Here's how the part is built. I have some questions about the finished solid (model axes, mm). Face numbers are marked on the shaded views. Give positions to 0.01 mm unless a question says otherwise; leave off trailing zeros. Loops run counter-clockwise (first coordinate to the right, second up) from the corner with the lowest first, then second, coordinate; pieces in that order, holes last.
Q1. Suppose I cut it at C-C (z = -36.5). Count the separate pieces of the cut face and the enclosed holes in it, and give its area (3 significant figures).
Q2. I need wall thicknesses on probe 1 along X at (y, z) = (-31, -40); probe 2 along X at (y, z) = (-8, -39); probe 3 along Z at (x, y) = (-44, -44.5). Which ranges of each line are inside material? Lowest first, please.
Q3. Suppose I cut it at A-A (y = -25). List the corners of the cut face in (x, z) for me.
Q4. Thinking about a two-plate mould opening in X: for the marked faces 1 and 2, which applies, pulls with the +X half, pulls with the -X half, needs draft (parallel to the pull), parting line crosses it, or undercut?
Q5. I'm going to push flat-ended pins straight in: P1, Ø2.5, axis at x = -2.5, y = -3, coming from the -Z side; P2, Ø4, axis at y = -17, z = -31.5, coming from the +X side; P3, Ø4, axis at x = 1.5, z = -1.5, coming from the -Y side. Where does each tip first touch, or does it pass through?
Q6. Suppose I cut it at B-B (x = -2). List the corners of the cut face in (y, z) for me, and give its area (3 significant figures).
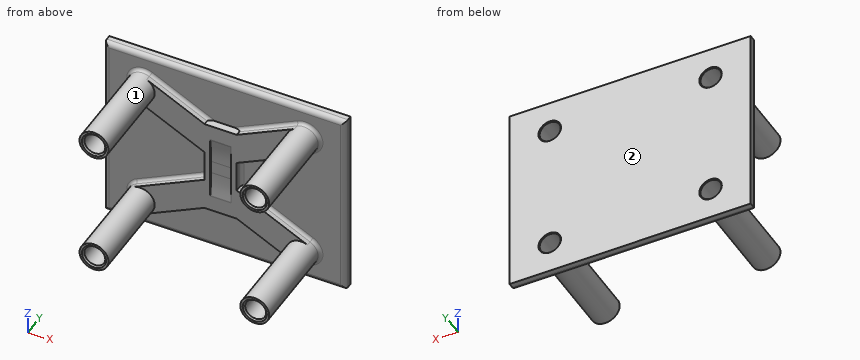
```python
from build123d import *

# Parameters (mm, degrees)
SKETCH_1_W          = 150
SKETCH_1_H          = 120
EXTRUDE_1_DEPTH     = 6
SKETCH_2_R          = 9
EXTRUDE_2_DEPTH     = 60
EXTRUDE_3_DEPTH     = 5
SKETCH_4_R          = 6.5
CUT_EXTRUDE_1_DEPTH = 117.537547597
CUT_EXTRUDE_2_DEPTH = 6.5
FILLET_1_R          = 2
FILLET_3_R          = 3
CHAMFER_1_SIZE      = 1
CHAMFER_2_SIZE      = 0.5


with BuildPart() as part:
    # 草图1 → 凸台-拉伸1 (new body)
    with BuildSketch(Plane(origin=(0, 0, 0), x_dir=(1, 0, 0), z_dir=(0, 1, 0))):
        Rectangle(SKETCH_1_W, SKETCH_1_H)
    extrude(amount=EXTRUDE_1_DEPTH)

    # 草图2 → 凸台-拉伸2 (add)
    with BuildSketch(Plane.XZ):
        with Locations(Location((-50, 40, 0), (0, 0, 90))):
            Circle(SKETCH_2_R)
        with Locations(Location((50, 40, 0), (0, 0, 90))):
            Circle(SKETCH_2_R)
        with Locations(Location((50, -40, 0), (0, 0, 90))):
            Circle(SKETCH_2_R)
        with Locations(Location((-50, -40, 0), (0, 0, 90))):
            Circle(SKETCH_2_R)
    extrude(amount=EXTRUDE_2_DEPTH)

    # 草图3 → 凸台-拉伸3 (add)
    with BuildSketch(Plane.XZ):
        with BuildLine():
            Line((-10, 30), (-45.963934166, 48.044263334))
            ThreePointArc((-45.963934166, 48.044263334), (-42.34086844, 44.726278002), (-41, 40))
            ThreePointArc((-41, 40), (-45.273721998, 32.34086844), (-54.036065834, 31.955736666))
            Line((-54.036065834, 31.955736666), (-10, 9.861425059))
            Line((-10, 9.861425059), (-10, -9.861425059))
            Line((-10, -9.861425059), (-54.036065834, -31.955736666))
            ThreePointArc((-54.036065834, -31.955736666), (-45.273721998, -32.34086844), (-41, -40))
            ThreePointArc((-41, -40), (-42.34086844, -44.726278002), (-45.963934166, -48.044263334))
            Line((-45.963934166, -48.044263334), (-10, -30))
            Line((-10, -30), (10, -30))
            Line((10, -30), (45.963934166, -48.044263334))
            ThreePointArc((45.963934166, -48.044263334), (41.955736666, -35.963934166), (54.036065834, -31.955736666))
            Line((54.036065834, -31.955736666), (10, -9.861425059))
            Line((10, -9.861425059), (10, 9.861425059))
            Line((10, 9.861425059), (54.036065834, 31.955736666))
            ThreePointArc((54.036065834, 31.955736666), (41.955736666, 35.963934166), (45.963934166, 48.044263334))
            Line((45.963934166, 48.044263334), (10, 30))
            Line((10, 30), (-10, 30))
        make_face()
    extrude(amount=EXTRUDE_3_DEPTH)

    # 草图4 → 切除-拉伸1 (cut, through all)
    with BuildSketch(Plane.XZ.offset(60)):
        with Locations(Location((-50, 40, 0), (0, 0, 270))):
            Circle(SKETCH_4_R)
        with Locations(Location((50, -40, 0), (0, 0, 270))):
            Circle(SKETCH_4_R)
        with Locations(Location((50, 40, 0), (0, 0, 270))):
            Circle(SKETCH_4_R)
        with Locations(Location((-50, -40, 0), (0, 0, 270))):
            Circle(SKETCH_4_R)
    extrude(amount=-CUT_EXTRUDE_1_DEPTH, mode=Mode.SUBTRACT)

    # 草图5 → 切除-拉伸2 (cut, symmetric)
    with BuildSketch(Plane(origin=(0, 0, 0), x_dir=(0, 0, -1), z_dir=(1, 0, 0))):
        with BuildLine():
            Line((-20, -5), (20, -5))
            ThreePointArc((20, -5), (12.023735411, -4.120233419), (4, -4))
            Line((4, -4), (-4, -4))
            ThreePointArc((-4, -4), (-12.023735411, -4.120233419), (-20, -5))
        make_face()
    extrude(amount=CUT_EXTRUDE_2_DEPTH, both=True, mode=Mode.SUBTRACT)

    # 圆角1
    fillet_1_edges = [part.edges().sort_by_distance(p)[0] for p in [
        (0, -5, -20),
        (0, -5, 20),
        (-58.044263334, 0, -44.036065834),
        (58.044263334, 0, -44.036065834),
        (-58.757807089, 0, 42.073840639),
        (58.757807089, 0, 42.073840639),
        (-27.981967083, 0, -39.022131667),
        (32.018032917, 0, -20.908580862),
        (27.981967083, 0, 39.022131667),
        (-32.018032917, 0, 20.908580862),
        (-10, 0, 0),
        (-32.018032917, 0, -20.908580862),
        (-27.981967083, 0, 39.022131667),
        (32.018032917, 0, 20.908580862),
        (10, 0, 0),
        (27.981967083, 0, -39.022131667),
    ]]
    fillet(fillet_1_edges, radius=FILLET_1_R)

    # 圆角3
    fillet_3_edges = [part.edges().sort_by_distance(p)[0] for p in [
        (0, 0, 60),
        (-75, 0, 0),
        (0, 0, -60),
        (75, 0, 0),
    ]]
    fillet(fillet_3_edges, radius=FILLET_3_R)

    # 倒角1
    chamfer_1_edges = [part.edges().sort_by_distance(p)[0] for p in [
        (-50, -60, -33.5),
        (50, -60, 46.5),
        (50, -60, -33.5),
        (-50, -60, 46.5),
    ]]
    chamfer(chamfer_1_edges, length=CHAMFER_1_SIZE)

    # 倒角2
    chamfer_2_edges = [part.edges().sort_by_distance(p)[0] for p in [
        (-50, 6, -33.5),
        (50, 6, 46.5),
        (50, 6, -33.5),
        (-50, 6, 46.5),
    ]]
    chamfer(chamfer_2_edges, length=CHAMFER_2_SIZE)


solid = part.part
```
Solutions:
1. separate pieces: 3
1. enclosed holes: 0
1. area: 1,630 mm2
2. probe 1: x = -59 to -56.5, -43.5 to -41, 41 to 43.5, 56.5 to 59
2. probe 2: x = -58.94 to -56.42, -43.58 to -41.06, 41.06 to 43.58, 56.42 to 58.94
2. probe 3: z = -46.71 to -42.5, -37.5 to -33.29, 33.29 to 37.5, 42.5 to 46.71
3. outline: circle Ø18 at (-50, -40); circle Ø18 at (-50, 40); circle Ø18 at (50, -40); circle Ø18 at (50, 40); hole circle Ø13 at (-50, -40); hole circle Ø13 at (-50, 40); hole circle Ø13 at (50, -40); hole circle Ø13 at (50, 40)
4. face 1: undercut
4. face 2: needs draft
5. P1: stops at z = -30
5. P2: stops at x = 56.22
5. P3: stops at y = -4
6. outline: (-5, -30) - (0, -30) - (0, -57) arc R3 ccw to (3, -60) - (6, -60) - (6, 60) - (3, 60) arc R3 ccw to (0, 57) - (0, 30) - (-5, 30) - (-5, 20.16) arc R2 ccw to (-4.98, 19.85) arc R84.62 cw to (-4, 4) - (-4, -4) arc R84.62 cw to (-4.98, -19.85) arc R2 ccw to (-5, -20.16) - close
6. area: 984 mm2
